from build123d import *

# Parameters (mm, degrees)
F1_DEPTH = 10
F2_R     = 1.1
F3_DEPTH = 6.2


with BuildPart() as f1:
    # F0 (on Front) → F1 (new body)
    with BuildSketch(Plane.XZ):
        Polygon((-5.35, 3), (-5.35, 0), (5.35, 0), (5.35, 3), (7.85, 3), (7.85, 6.2), (-7.85, 6.2), (-7.85, 3), align=None)
    extrude(amount=F1_DEPTH)

    # F2 (on face) → F3 (cut, through all)
    with BuildSketch(Plane.XY.offset(6.2)):
        with Locations((0, -5)):
            Circle(F2_R)
    extrude(amount=-F3_DEPTH, mode=Mode.SUBTRACT)


solid = f1.part
For this review, take the finished solid that the model builds, in its own axes (mm). A direction names the side the tool comes from. Coordinates: 2 decimals unless noted, no trailing zeros. Order: outer loops, then holes, each group sorted by start corner. A loop starts at its lowest first (then second) coordinate and runs counter-clockwise, first axis right, second up. Notation, with made-up numbers: (82.25, 1.5) - (106.25, 1.5) arc R11 ccw to (106.25, 6.5) - close; hole circle Ø1 at (85, 61). An arc over 180 degrees is marked (long way). Answer as CSV lines item,"result". Start each with the question number.
1) Insertion check: P1, Ø1.3, axis at x = 0, y = -5, coming from the +Z side; P2, Ø2.5, axis at y = -3, z = 1, coming from the -X side; P3, Ø1.5, axis at y = -3, z = 1, coming from the +X side; P4, Ø2, axis at x = 6.5, y = -4.5, coming from the -Z side. Each pin has a flat end and moves straight along its axis. Give the tip position at first contact, or say it passes through.
2) Add section B-B (y = -5). State the section outline as (x, z) points.
3) To check wall thickness, follow line 1 along Y through (x, z) = (0, 3.75); line 2 along X through (y, z) = (-3.5, 2.75); line 3 along Z through (x, y) = (6.75, -6.75). State the ranges of each line that lie inside material, in increasing order. Write a range as [from, to].
4) Draft analysis for pull direction X (two halves, no side actions). For faces 1 (the cylindrical face through (0.59, -4.07, 3.14)), 2 (the flat face through (0, -10, 3)), 3 (the flat face through (5.35, -5, 1)), state which applies: +X half, -X half, draft (parallel to the pull), parting line (faces both ways), or undercut.
5) Machinability: for faces 4 (the flat face through (-1.3, -4.9, 0)), 5 (the flat face through (7, -5, 3)), 6 (the flat face through (-7, -5, 3)), which of the approach directions +Z, -Z, +X, -X, +Y, -Y give a long, thin tool a straight path to every point of the face, cutting with its end or side? Answer none if there is none.
6) Add section A-A (x = 0). State the section outline as (y, z) points.
7) Add section C-C (z = 2.5). State the section outline as (x, y) points, then the cut area to 3 significant figures.
8) Add section D-D (y = -3). State the section outline as (x, z) points, then the cut area to 3 significant figures.
Result:
1,P1,"through"
1,P2,"x = -5.35"
1,P3,"x = 5.35"
1,P4,"z = 3"
2,outline,"(-7.85, 3) - (-5.35, 3) - (-5.35, 0) - (-1.1, 0) - (-1.1, 6.2) - (-7.85, 6.2) - close; (1.1, 0) - (5.35, 0) - (5.35, 3) - (7.85, 3) - (7.85, 6.2) - (1.1, 6.2) - close"
3,line 1,"[-10, -6.1], [-3.9, 0]"
3,line 2,"[-5.35, 5.35]"
3,line 3,"[3, 6.2]"
4,face 1,"undercut"
4,face 2,"draft"
4,face 3,"+X half"
5,face 4,"-Z, +X, -X, +Y, -Y"
5,face 5,"-Z, +X, +Y, -Y"
5,face 6,"-Z, -X, +Y, -Y"
6,outline,"(-10, 0) - (-6.1, 0) - (-6.1, 6.2) - (-10, 6.2) - close; (-3.9, 0) - (0, 0) - (0, 6.2) - (-3.9, 6.2) - close"
7,outline,"(-5.35, -10) - (5.35, -10) - (5.35, 0) - (-5.35, 0) - close; hole circle Ø2.2 at (0, -5)"
7,area,"103 mm^2"
8,outline,"(-7.85, 3) - (-5.35, 3) - (-5.35, 0) - (5.35, 0) - (5.35, 3) - (7.85, 3) - (7.85, 6.2) - (-7.85, 6.2) - close"
8,area,"82.3 mm^2"
